```python
from build123d import *

# Parameters (mm, degrees)
BOSS_EXTRUDE1_DEPTH             = 5
BOSS_EXTRUDE2_REACH             = 19.804
BOSS_EXTRUDE2_DIRECTION_2_REACH = 19.804
BOSS_EXTRUDE3_DEPTH             = 2
SKETCH4_R                       = 2.65
CUT_EXTRUDE1_DEPTH              = 29.091194779
SKETCH9_W                       = 64.865756982
SKETCH9_H                       = 28.956889813
CUT_EXTRUDE2_DEPTH              = 32.5
CUT_EXTRUDE3_DEPTH              = 29.618053883
CHAMFER3_SIZE                   = 3
CHAMFER3_SIZE_2                 = 4.914912266


with BuildPart() as part:
    # Sketch2 → Boss-Extrude1 (new, symmetric)
    with BuildSketch(Plane.XY):
        with BuildLine():
            Line((-10, 6), (10, 6))
            ThreePointArc((10, 6), (16, 0), (10, -6))
            Line((10, -6), (-10, -6))
            ThreePointArc((-10, -6), (-16, 0), (-10, 6))
        make_face()
    extrude(amount=BOSS_EXTRUDE1_DEPTH, both=True)

    # Boss-Extrude2: up to this face of the body (flat: up to its plane)
    boss_extrude2_end = Plane(part.part.faces().sort_by_distance((0, 6, 0))[0])
    # Sketch3 → Boss-Extrude2 (add, up to the picked face)
    with BuildSketch(Plane(origin=(0, 0, 0), x_dir=(1, 0, 0), z_dir=(0, 1, 0)), mode=Mode.PRIVATE) as boss_extrude2_sk1:
        Polygon((-5, 5), (-5, 9.823085464), (13, 5), align=None)
    boss_extrude2_tool1 = split(extrude(boss_extrude2_sk1.sketch, amount=BOSS_EXTRUDE2_REACH, mode=Mode.PRIVATE), bisect_by=boss_extrude2_end, keep=Keep.BOTH, mode=Mode.PRIVATE)
    # Sketch3 → Boss-Extrude2 (add, up to the picked face)
    with BuildSketch(Plane(origin=(0, 0, 0), x_dir=(1, 0, 0), z_dir=(0, 1, 0)), mode=Mode.PRIVATE) as boss_extrude2_sk2:
        Polygon((-11, -5), (7, -9.823085464), (7, -5), align=None)
    boss_extrude2_tool2 = split(extrude(boss_extrude2_sk2.sketch, amount=BOSS_EXTRUDE2_REACH, mode=Mode.PRIVATE), bisect_by=boss_extrude2_end, keep=Keep.BOTH, mode=Mode.PRIVATE)
    add(boss_extrude2_tool1.solids().sort_by(Axis((1, 0, -6.607695), (0, 1, 0)))[0])
    add(boss_extrude2_tool2.solids().sort_by(Axis((1, 0, 6.607695), (0, 1, 0)))[0])

    # Boss-Extrude2 direction 2: up to this face of the body (flat: up to its plane)
    boss_extrude2_direction_2_end = Plane(part.part.faces().sort_by_distance((0, -6, 0))[0])
    # Sketch3 → Boss-Extrude2 direction 2 (add, up to the picked face)
    with BuildSketch(Plane(origin=(0, 0, 0), x_dir=(1, 0, 0), z_dir=(0, 1, 0)), mode=Mode.PRIVATE) as boss_extrude2_direction_2_sk1:
        Polygon((-5, 5), (-5, 9.823085464), (13, 5), align=None)
    boss_extrude2_direction_2_tool1 = split(extrude(boss_extrude2_direction_2_sk1.sketch, amount=-BOSS_EXTRUDE2_DIRECTION_2_REACH, mode=Mode.PRIVATE), bisect_by=boss_extrude2_direction_2_end, keep=Keep.BOTH, mode=Mode.PRIVATE)
    # Sketch3 → Boss-Extrude2 direction 2 (add, up to the picked face)
    with BuildSketch(Plane(origin=(0, 0, 0), x_dir=(1, 0, 0), z_dir=(0, 1, 0)), mode=Mode.PRIVATE) as boss_extrude2_direction_2_sk2:
        Polygon((-11, -5), (7, -9.823085464), (7, -5), align=None)
    boss_extrude2_direction_2_tool2 = split(extrude(boss_extrude2_direction_2_sk2.sketch, amount=-BOSS_EXTRUDE2_DIRECTION_2_REACH, mode=Mode.PRIVATE), bisect_by=boss_extrude2_direction_2_end, keep=Keep.BOTH, mode=Mode.PRIVATE)
    add(boss_extrude2_direction_2_tool1.solids().sort_by(Axis((1, 0, -6.607695), (0, -1, 0)))[0])
    add(boss_extrude2_direction_2_tool2.solids().sort_by(Axis((1, 0, 6.607695), (0, -1, 0)))[0])

    # Sketch8 → Boss-Extrude3 (add)
    with BuildSketch(Plane.XY.offset(5)):
        with BuildLine():
            Line((-10, 8.5), (10, 8.5))
            ThreePointArc((10, 8.5), (18.5, 0), (10, -8.5))
            Line((10, -8.5), (-10, -8.5))
            ThreePointArc((-10, -8.5), (-18.5, 0), (-10, 8.5))
        make_face()
    boss_extrude3 = extrude(amount=-BOSS_EXTRUDE3_DEPTH)

    # Mirror1: Boss-Extrude3 across plane
    add(boss_extrude3.mirror(Plane.XY))

    # Sketch4 → Cut-Extrude1 (cut, through all)
    with BuildSketch(Plane(origin=(-1.986860279, 0, 7.415063509), x_dir=(0.96592582628907, 0, 0.25881904510251436), z_dir=(-0.25881904510251436, 0, 0.96592582628907))):
        with Locations((2.303882384, 0)):
            Circle(SKETCH4_R)
    extrude(amount=-CUT_EXTRUDE1_DEPTH, mode=Mode.SUBTRACT)

    # Sketch9 → Cut-Extrude2 (cut, symmetric)
    with BuildSketch(Plane(origin=(0, 0, 0), x_dir=(1, 0, 0), z_dir=(0, 1, 0))):
        with Locations((0.241735823, 14.478444907)):
            Rectangle(SKETCH9_W, SKETCH9_H)
    extrude(amount=CUT_EXTRUDE2_DEPTH, both=True, mode=Mode.SUBTRACT)

    # Sketch10 → Cut-Extrude3 (cut, through all)
    with BuildSketch(Plane(origin=(7, 0, 0), x_dir=(0, 0, -1), z_dir=(1, 0, 0))):
        Polygon((-5, 6), (-9.823085464, 1), (-9.823085464, -1), (-5, -6), (-15.161694792, -6), (-15.161694792, 6), align=None)
    extrude(amount=-CUT_EXTRUDE3_DEPTH, mode=Mode.SUBTRACT)

    # Chamfer3
    # the kernel refuses this chamfer: 4.914912266, 3 mm, written as the material it takes off along each edge
    with BuildSketch(Plane(origin=(7, 13.693017634, 9.823085464), x_dir=(-0.9797390561393613, 0, -0.2002782611147635), z_dir=(0, -1, 0))) as chamfer3_piece_1_section:
        Polygon((CHAMFER3_SIZE * 0.998191085646, CHAMFER3_SIZE * 0.0601211821046), (CHAMFER3_SIZE_2 * 0.200278261104, CHAMFER3_SIZE_2 * 0.979739056086), (0, 0), align=None)
    chamfer3_piece_1 = extrude(amount=27.386035267, mode=Mode.PRIVATE)
    chamfer3_piece_1 = split(chamfer3_piece_1, bisect_by=Plane(origin=(6.06140933, 0, 5), z_dir=(0, 0, 1)), keep=Keep.TOP, mode=Mode.PRIVATE)
    add(chamfer3_piece_1, mode=Mode.SUBTRACT)


solid = part.part
```
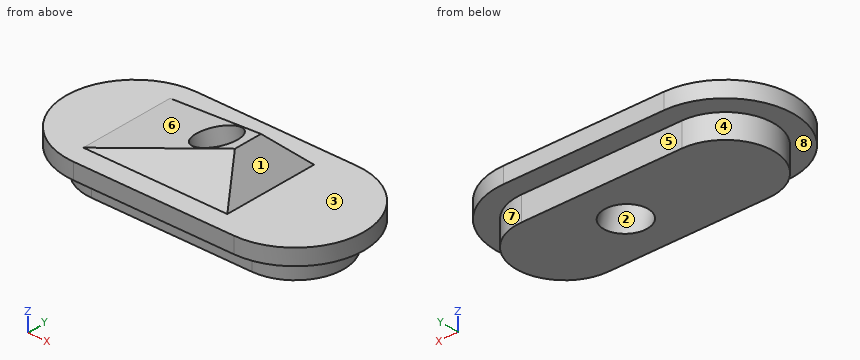
Geometry check sheet. Reference: the model listing, model coordinates, mm. Face numbers are marked on the shaded views. A direction names the side the tool comes from. Give positions to 0.01 mm unless a question says otherwise; leave off trailing zeros. Loops run counter-clockwise (first coordinate to the right, second up) from the corner with the lowest first, then second, coordinate; pieces in that order, holes last. Notation, with made-up numbers: M -39,2 L 10,2 A11 ccw 10,20 Z; hole C -31,-28.5 d9. An arc over 180 degrees is marked long. Write item = value, one per line. Start each with the question number.
1. Section check B-B, the plane x = 8. Enter the section's corners in (y, z).
2. Thickness scan on probe 1 along Z at (x, y) = (7, -2.25); probe 2 along Z at (x, y) = (15.5, -4); probe 3 along Y at (x, z) = (3, 6.5). Record the ranges inside material, lowest first.
3. Draft check along X on the marked faces 1, 2 and 3. Enter one of: +X half, -X half, draft (parallel to the pull), parting line (faces both ways), or undercut.
4. Section check D-D, the plane x = -5. Enter the section's corners in (y, z), plus the area to 3 significant figures.
5. Tool access check on the marked faces 4, 5, 6, 7 and 8. Record the directions out of +Z, -Z, +X, -X, +Y, -Y that give a thin tool (end or side, any length) a straight path to the whole face; none if there is none.
6. Section check C-C, the plane y = 5. Enter the section's corners in (x, z), plus the area to 3 significant figures.
7. Go/stop test with flat-tipped pins: P1, Ø5, axis at y = 1.5, z = 3, coming from the +X side; P2, Ø4, axis at y = 4, z = 1.5, coming from the -X side; P3, Ø1.5, axis at x = -14, z = 1, coming from the +Y side; P4, Ø5, axis at x = -3, y = -3.5, coming from the +Z side. Record where each tip stops, or that it passes through.
8. Section check A-A, the plane y = 0. Enter the section's corners in (x, z).
Values follow:
q1.outline = M -8.5,3 L -6,3 L -6,0 L 6,0 L 6,3 L 8.5,3 L 8.5,5 L -8.5,5 Z
q2.probe_1 = 0 to 5
q2.probe_2 = 3 to 5
q2.probe_3 = -4.44 to -1.36, 1.36 to 4.44
q3.face_1 = +X half
q3.face_2 = undercut
q3.face_3 = draft
q4.outline = M -8.5,3 L -6,3 L -6,0 L 6,0 L 6,3 L 8.5,3 L 8.5,5 L 6,5 L 4.33,6.61 L -4.33,6.61 L -6,5 L -8.5,5 Z
q4.area = 86.6 mm^2
q5.face_4 = -Z, -X
q5.face_5 = -Z, +X, -X, +Y
q5.face_6 = +Z, -X, +Y, -Y
q5.face_7 = -Z, +X
q5.face_8 = -Z
q6.outline = M -16.87,3 L -13.32,3 L -13.32,0 L 13.32,0 L 13.32,3 L 16.87,3 L 16.87,5 L 6.94,5 L 6.26,5.96 L -7.4,5.96 L -11,5 L -16.87,5 Z
q6.area = 163 mm^2
q7.P1 = 18.5
q7.P2 = -18.07
q7.P3 = 5.04
q7.P4 = 7.8
q8.outline = M -18.5,3 L -16,3 L -16,0 L -0.36,0 L -2.32,7.33 L -11,5 L -18.5,5 Z; M 2.8,8.7 L 5.13,0 L 16,0 L 16,3 L 18.5,3 L 18.5,5 L 6.94,5 L 4.1,9.05 Z
